Autodesk Fusion 360 part; units mm, degrees
sketch "Adapter Sketch" plane through (0, 0, 0) normal (0, 0, 1) x (1, 0, 0)
  circle A0 centre (0, 0) radius 25.25
  circle A1 centre (0, 0) radius 29
  circle A2 centre (0, 0) radius 24
  line L0 (25.0221, -14.4721) -> (0.0222, 28.9059)
  line L1 (0.0222, 28.9059) -> (-25.0443, -14.4337)
  line L2 (-25.0443, -14.4337) -> (25.0221, -14.4721)
  dimension "d1" = 50.5
  dimension "d2" = 58
  dimension "d3" = 48
extrude "Extrude1" add sketch "Adapter Sketch" along normal blind 1 contours A0 A2 L0 | A0 A2 L0 L1 | A0 A2 L0 L2 | A0 A2 L1 | A0 A2 L2 | A0 A2 L1 L2
extrude "Extrude2" add sketch "Adapter Sketch" along normal blind 40 contours A0 L0 L1 | A0 L0 L2 | A0 L1 L2 | A1
hole "Hole1" at (25.6055, -13.6147, 35.9754) direction (-0.8829, 0.4695, 0) diameter 4 depth 5 tip angle 180
hole "Hole2" at (-25.1147, -14.5, 35.7941) direction (0.866, 0.5, 0) diameter 4 depth 5 tip angle 180
hole "Hole3" at (0, 29, 36.074) direction (0, -1, 0) diameter 4 depth 5 tip angle 180
The listing builds one solid part. Answer for the finished solid, in the listing's coordinates (mm). A direction names the side the tool comes from. Give positions to 0.01 mm unless a question says otherwise; leave off trailing zeros. Order: outer loops, then holes, each group sorted by start corner. A loop starts at its lowest first (then second) coordinate and runs counter-clockwise, first axis right, second up. Notation, with made-up numbers: M 75.5,-17 L 93.5,-17 A15 cw 93.5,8 Z; hole C 74,86 d5. An arc over 180 degrees is marked long. Put each result on its own line as item: value. Start each with the question number.
Item 1: Which of the six approach directions +Z, -Z, +X, -X, +Y, -Y give full straight-line access (tool end or side, diameter ignored) to faces 1 (the face through (-5.47, 24.65, 20.23)), 2 (the face through (-0.088, 27.059, 34.076)), 3 (the face through (24.251, -12.027, 34.128))?
Item 2: The part is cut by section A-A, the plane y = 0. Determine the outline of the cut face in (x, z).
Item 3: Flat-ended cylindrical pins translate along their axes: P1, Ø1, axis at x = -3.5, z = 36, coming from the +Y side; P2, Ø5, axis at x = -18, y = -7, coming from the +Z side; P3, Ø6, axis at x = -9, z = 10.5, coming from the +Y side; P4, Ø8, axis at y = -21.5, z = 35, coming from the +X side. Find the tip coordinate at first contact, or state that the pin passes through.
Item 4: The part is cut by section C-C, the plane x = 7. Determine the outline of the cut face in (y, z), and give its area (3 significant figures).
Item 5: For a pull along X with two mould halves and no side action, classify faces 4 (the face through (22.33, -9.23, 1)), 5 (the face through (13.38, 25.73, 19.72)), 6 (the face through (-9, 24, 40)) as +X half, -X half, draft (parallel to the pull), parting line (faces both ways), or undercut.
Item 6: The part is cut by section B-B, the plane x = 0. Determine the outline of the cut face in (y, z), and give its area (4 significant figures).
Item 7: Find the intervals of material crossed by line 1 along Y through (x, z) = (0, 0.65); line 2 along Z through (x, y) = (0, 26); line 3 along Y through (x, z) = (0, 30), in increasing order.
Item 8: The part is cut by section D-D, the plane z = 27.5. Determine the outline of the cut face in (x, y), and give its area (3 significant figures).
Answer key:
1. face 1: +Z
1. face 2: +Y
1. face 3: none
2. outline: M -29,0 L -24,0 L -24,1 L -25.25,1 L -25.25,40 L -29,40 Z; M 24,0 L 29,0 L 29,40 L 25.25,40 L 25.25,1 L 24,1 Z
3. P1: stops at y = 28.84
3. P2: passes through
3. P3: stops at y = 28.37
3. P4: stops at x = 23.12
4. outline: M -28.14,0 L -22.96,0 L -22.96,1 L -24.26,1 L -24.26,40 L -28.14,40 Z; M 22.96,0 L 28.14,0 L 28.14,40 L 24.26,40 L 24.26,1 L 22.96,1 Z
4. area: 313 mm²
5. face 4: undercut
5. face 5: parting line
5. face 6: draft
6. outline: M -29,0 L -24,0 L -24,1 L -25.25,1 L -25.25,40 L -29,40 Z; M 24,0 L 29,0 L 29,34.07 L 25.25,34.07 L 25.25,1 L 24,1 Z; M 25.25,38.07 L 29,38.07 L 29,40 L 25.25,40 Z
6. area: 287.5 mm²
7. line 1: y = -29 to -24, 24 to 29
7. line 2: z = 0 to 34.07, 38.07 to 40
7. line 3: y = -29 to -25.25, 25.25 to 29
8. outline: C 0,0 d58; hole C 0,0 d50.5
8. area: 639 mm²
